Geometry: final body of the model. Coordinates: model frame, mm. Give positions to 0.01 mm unless a question says otherwise; leave off trailing zeros. Order: outer loops, then holes, each group sorted by start corner. A loop starts at its lowest first (then second) coordinate and runs counter-clockwise, first axis right, second up. Notation, with made-up numbers: (84, 55) -> (139, 55) arc R17 cw to (139, 78) -> close; hole circle Ø3 at (47.25, -32). An arc over 180 degrees is marked (long way). Write item = value, one per line.
Autodesk Inventor part; units mm, degrees
ref_plane "YZ Plane" through (0, 0, 0) normal (1, 0, 0) x (0, 1, 0)
ref_plane "XZ Plane" through (0, 0, 0) normal (0, 1, 0) x (-1, 0, 0)
ref_plane "XY Plane" through (0, 0, 0) normal (0, 0, 1) x (1, 0, 0)
sketch "スケッチ1" plane through (0, 0, 0) normal (0, 0, 1) x (1, 0, 0)
  line L0 (-25, -25) -> (25, -25)
  line L1 (25, -25) -> (25, 25)
  line L2 (25, 25) -> (-25, 25)
  line L3 (-25, 25) -> (-25, -25)
  line L4 (-25, -25) -> (25, 25) construction
  line L5 (25, -25) -> (-25, 25) construction
  point P0 (0, 0)
  dimension "d0" = 50
  dimension "d1" = 50
extrude "押し出し1" add sketch "スケッチ1" along normal blind 7.5
sketch "スケッチ2" plane through (0, 0, 7.5) normal (0, 0, 1) x (1, 0, 0)
  line L0 (-25, 25) -> (-25, -25)
  line L1 (-25, -25) -> (25, -25)
  point P0 (0, 0)
  point P1 (-15, 12.836)
  point P2 (9, 12.836)
  point P3 (9, -17.164)
  point P4 (-15, -17.164)
  dimension "d4" = 10
  dimension "d5" = 10
  dimension "d6" = 30
  dimension "d7" = 30
  dimension "d8" = 24
  dimension "d16" = 7.836
  dimension "d17" = 7.836
hole "穴1" at (-15, 12.836, 7.5) at (9, 12.836, 7.5) at (9, -17.164, 7.5) at (-15, -17.164, 7.5) direction (0, 0, -1) diameter 3.4 end through all
properties part number "20220509_知能ロボットキャスタ"
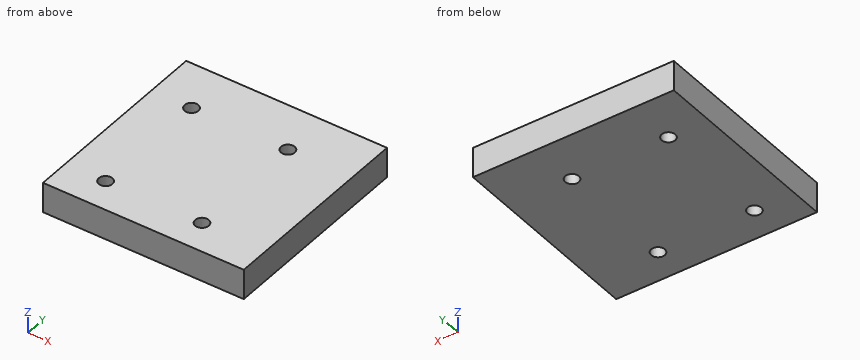
1) Section query A-A (x = 9). Output: boundary loops of the cut face in (y, z), plus the area to 3 significant figures.
Check sheet entries:
outline = (-25, 0) -> (-18.86, 0) -> (-18.86, 7.5) -> (-25, 7.5) -> close; (-15.46, 0) -> (11.14, 0) -> (11.14, 7.5) -> (-15.46, 7.5) -> close; (14.54, 0) -> (25, 0) -> (25, 7.5) -> (14.54, 7.5) -> close
area = 324 mm²
2) Line query: line 1 (Y direction, x = -15, z = 2); line 2 (X direction, y = 13, z = 4.5). Output: solid intervals per line, ascending. Write a range as from..to.
Check sheet entries:
line_1 = -25..-18.86, -15.46..11.14, 14.54..25
line_2 = -25..-16.69, -13.31..7.31, 10.69..25
3) First-contact query: P1, Ø2, axis at x = -15, y = -17.164, coming from the +Z side. Flat tip, straight axial feed; report the tip coordinate or a pass-through.
Check sheet entries:
P1 = through
